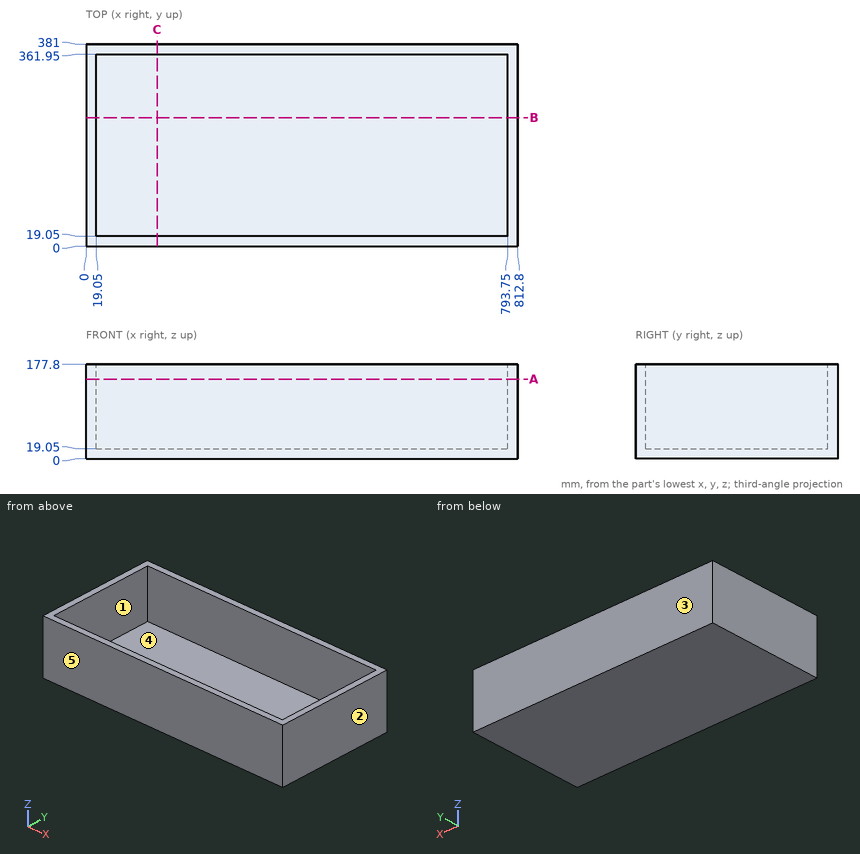
Job drawing, mm, ordinate dimensions from the low corner. One solid piece. A direction names the side the tool comes from. Coordinates: 2 decimals unless noted, no trailing zeros. Order: outer loops, then holes, each group sorted by start corner. A loop starts at its lowest first (then second) coordinate and runs counter-clockwise, first axis right, second up. Notation, with made-up numbers: M 5,83 L 51,83 A19 ccw 51,96 Z; hole C 52,68 d5. An arc over 180 degrees is marked long. One line per question, with ' | ' between items.
Q1. Slice it at B-B (y = 242.5). Give the cut face in (x, z), and give its area (3 significant figures).
A:
outline: M 0,0 L 812.8,0 L 812.8,177.8 L 793.75,177.8 L 793.75,19.05 L 19.05,19.05 L 19.05,177.8 L 0,177.8 Z | area: 21,500 mm^2
Q2. Slice it at C-C (x = 134). Give the cut face in (y, z).
A:
outline: M 0,0 L 381,0 L 381,177.8 L 361.95,177.8 L 361.95,19.05 L 19.05,19.05 L 19.05,177.8 L 0,177.8 Z
Q3. Drill centre lines: line 1 (X direction, y = 119.5, z = 44); line 2 (Y direction, x = 134, z = 137); line 3 (Z direction, x = 299, y = 78). Where is each one in solid material? Low to high.
A:
line 1: x = 0 to 19.05, 793.75 to 812.8 | line 2: y = 0 to 19.05, 361.95 to 381 | line 3: z = 0 to 19.05
Q4. 3-axis set-ups, long thin cutter, end or side, ignore diameter. For the marked faces 4 and 5: which of +Z, -Z, +X, -X, +Y, -Y reach the whole face in a straight line?
A:
face 4: +Z | face 5: +Z, -Z, +X, -X, -Y
Q5. Two-plate mould, pull along X, no slides. Class the marked faces 1, 2 and 3: +X half, -X half, draft (parallel to the pull), parting line (faces both ways), or undercut.
A:
face 1: undercut | face 2: +X half | face 3: draft
Q6. Pin check, flat tips, straight feed: P1, Ø3, axis at x = 236, y = 274, coming from the +Z side; P2, Ø1, axis at x = 226, z = 150, coming from the -Y side. Stop position of each tip, or through.
A:
P1: stops at z = 19.05 | P2: stops at y = 0
Q7. Slice it at A-A (z = 150). Give the cut face in (x, y).
A:
outline: M 0,0 L 812.8,0 L 812.8,381 L 0,381 Z; hole M 19.05,19.05 L 793.75,19.05 L 793.75,361.95 L 19.05,361.95 Z
